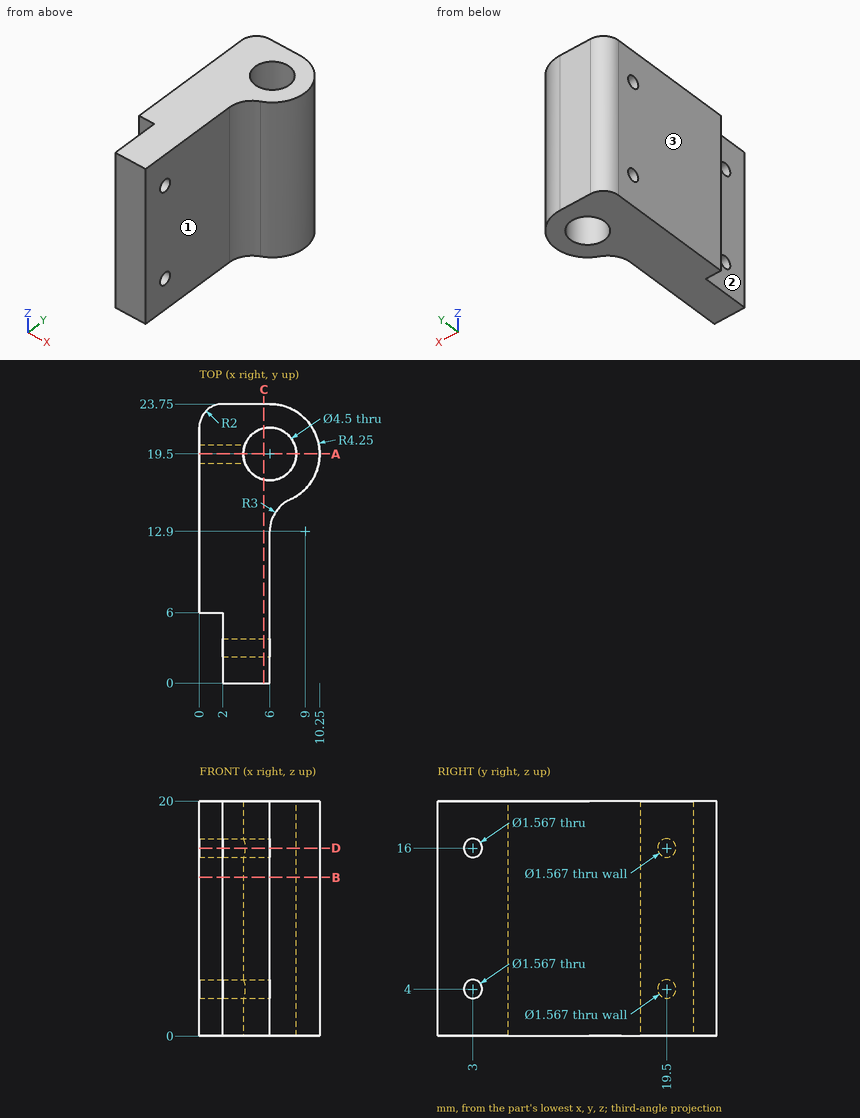
Design review of the part shown in the three views and the two pictorial views. Dimensions are in mm from the part's minimum x, y and z. A direction names the side the tool comes from. Give positions to 0.01 mm unless a question says otherwise; leave off trailing zeros. Write each loop counter-clockwise with the first axis right and the second up, starting at its lowest first coordinate (ties: lowest second). Pieces come first, ordered by that corner, then holes. Notation, with made-up numbers: M 0.5,62.25 L 36.5,62.25 A34 cw 36.5,95.25 Z; hole C 54.25,89 d4. An arc over 180 degrees is marked long. Answer as CSV lines item,"result".
1. Consider section A-A, the plane y = 19.5. Write out the cut boundary in (x, z), then the cut area to 3 significant figures.
Findings:
outline,"M 0,0 L 3.75,0 L 3.75,3.22 L 0,3.22 Z; M 0,4.78 L 3.75,4.78 L 3.75,15.22 L 0,15.22 Z; M 0,16.78 L 3.75,16.78 L 3.75,20 L 0,20 Z; M 8.25,0 L 10.25,0 L 10.25,20 L 8.25,20 Z"
area,"103 mm2"
2. Consider section B-B, the plane z = 13.5. Write out the cut boundary in (x, y).
Findings:
outline,"M 0,6 L 2,6 L 2,0 L 6,0 L 6,12.9 A3 cw 7.76,15.63 A4.25 ccw 6,23.75 L 2,23.75 A2 ccw 0,21.75 Z; hole C 6,19.5 d4.5"
3. Consider section C-C, the plane x = 5.5. Write out the cut boundary in (y, z).
Findings:
outline,"M 0,0 L 17.31,0 L 17.31,20 L 0,20 Z; M 21.69,0 L 23.75,0 L 23.75,20 L 21.69,20 Z; hole C 3,4 d1.57; hole C 3,16 d1.57"
4. Consider section D-D, the plane z = 16. Write out the cut boundary in (x, y), then the cut area to 3 significant figures.
Findings:
outline,"M 0,6 L 2,6 L 2,3.78 L 6,3.78 L 6,12.9 A3 cw 7.76,15.63 A4.25 ccw 6,23.75 L 2,23.75 A2 ccw 0,21.75 L 0,20.28 L 3.89,20.28 A2.25 cw long 3.89,18.72 L 0,18.72 Z; M 2,0 L 6,0 L 6,2.22 L 2,2.22 Z"
area,"131 mm2"
5. For the marked faces 1, 2 and 3, list the 3-axis set-ups (+Z, -Z, +X, -X, +Y, -Y) from which the entire face can be reached by the end or side of a thin tool; tool diameter is ignored.
Findings:
face 1,"+Z, -Z, +X, -Y"
face 2,"+Z, -Z, -X, -Y"
face 3,"+Z, -Z, -X, +Y, -Y"
6. For pin 1 (1.4 mm diameter, centred on y = 19.5, z = 16, fed in from -X); pin 2 (1 mm diameter, centred on x = 0.5, z = 7.5, fed in from -Y); pin 3 (4 mm diameter, centred on y = 7, z = 7.5, fed in from +X), all flat-tipped, find the tip position at first contact; note any pin that passes through.
Findings:
pin 1,"stops at x = 8.14"
pin 2,"stops at y = 6"
pin 3,"stops at x = 6"
7. Wall thickness on line 1 (Y direction, x = 3.5, z = 16); line 2 (Z direction, x = 3.1, y = 3); line 3 (X direction, y = 19.5, z = 9): over which ranges is each line inside the solid? List them lowest first.
Findings:
line 1,"y = 0 to 2.22, 3.78 to 18.72, 20.28 to 23.75"
line 2,"z = 0 to 3.22, 4.78 to 15.22, 16.78 to 20"
line 3,"x = 0 to 3.75, 8.25 to 10.25"
